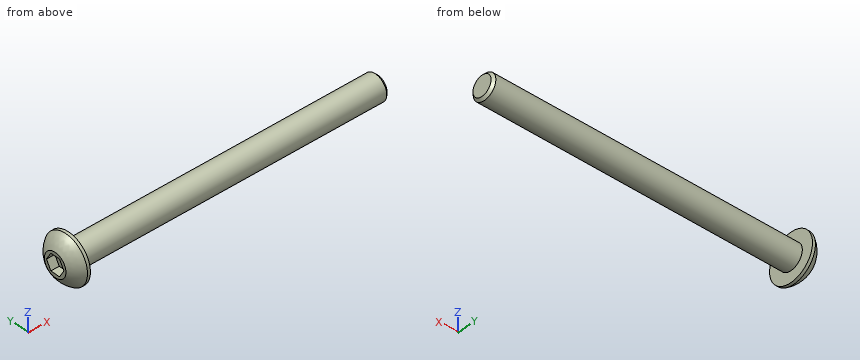
```python
from build123d import *

# Parameters (mm, degrees)
CHAMFER1_SIZE      = 0.3
CUT_EXTRUDE1_DEPTH = 1
SCALE1_SCALE       = 1.667


with BuildPart() as part:
    # Sketch1 → Revolve1 (revolve)
    with BuildSketch(Plane.XY):
        with BuildLine():
            Line((38.65, 0), (0, 0))
            Line((0, 0), (0, 1.425))
            ThreePointArc((0, 1.425), (0.549895392, 2.228823502), (1.3, 2.85))
            Line((1.3, 2.85), (1.65, 2.85))
            Line((1.65, 2.85), (1.65, 1.5))
            Line((1.65, 1.5), (38.65, 1.5))
            Line((38.65, 1.5), (38.65, 0))
        make_face()
    revolve(axis=Axis((38.65, 0, 0), (-1, 0, 0)))

    # Chamfer1
    chamfer1_edges = [part.edges().sort_by_distance(p)[0] for p in [
        (38.65, -1.5, 0),
    ]]
    chamfer(chamfer1_edges, length=CHAMFER1_SIZE)

    # Sketch2 → Cut-Extrude1 (cut)
    with BuildSketch(Plane.ZY):
        Polygon((0, 1.154700538), (-1, 0.577350269), (-1, -0.577350269), (0, -1.154700538), (1, -0.577350269), (1, 0.577350269), align=None)
    extrude(amount=-CUT_EXTRUDE1_DEPTH, mode=Mode.SUBTRACT)


with BuildPart() as part_1:
    # Scale1: scaled about (18.321522069, 0, 0)
    add(part.part.scale(SCALE1_SCALE).moved(Location((-12.22045522, 0, 0))))


solid = part_1.part
```
Build history of the part. All positions in model axes, mm. Coordinates: 2 decimals unless noted, no trailing zeros. Order: outer loops, then holes, each group sorted by start corner. A loop starts at its lowest first (then second) coordinate and runs counter-clockwise, first axis right, second up. Notation, with made-up numbers: M -36,22.5 L 5,22.5 A23 ccw 5,30.5 Z; hole C 45,-29.5 d11. An arc over 180 degrees is marked long. One line per question, with ' | ' between items. Start each with the question number.
1. Cut at A-A (x = 10). Write the cut outline in (y, z), plus the area to 3 significant figures.
2. Wall check: line 1 along X through (y, z) = (0.5, 0.75); line 2 along Y through (x, z) = (42.5, 0). Give the ranges that are in metal, low to high. Write a range as [from, to].
3. Flat gauge pins, fed straight in: P1, Ø5, axis at x = 2.5, y = -2.5, coming from the +Z side; P2, Ø4, axis at x = 35.5, z = 0, coming from the -Y side; P3, Ø4, axis at x = -2, y = -2.5, coming from the -Z side. Where does each tip first touch, or does it go through?
The answers:
1) outline: C 0,0 d5 | area: 19.6 mm2
2) line 1: x = [-10.55, 52.21] | line 2: y = [-2.5, 2.5]
3) P1: stops at z = 2.5 | P2: stops at y = -2.5 | P3: stops at z = -2.45
